```python
from build123d import *

# Parameters (mm, degrees)
F1_DEPTH = 5
F2_DEPTH = 4
F3_DEPTH = 4
F4_R     = 3.22905
F4_R_2   = 3.229051
F5_DEPTH = 25


with BuildPart() as f1:
    # F0 (on Top) → F1 (new body)
    with BuildSketch(Plane.XY):
        Polygon((16.577804, 72.764611), (3.665576, 72.739941), (-9.246652, 72.715272), (-9.147654, 20.899711), (3.838721, 20.904658), (10.953161, 20.92936), (10.913751, 41.556355), (16.625739, 47.675223), align=None)
    extrude(amount=F1_DEPTH)

    # F0 (on Top) → F2 (join)
    with BuildSketch(Plane.XY):
        Polygon((16.577804, 72.764611), (3.665576, 72.739941), (-9.246652, 72.715272), (-9.147654, 20.899711), (3.838721, 20.904658), (10.953161, 20.92936), (10.913751, 41.556355), (16.625739, 47.675223), align=None)
    extrude(amount=F2_DEPTH)

    # F0 (on Top) → F3 (join)
    with BuildSketch(Plane.XY):
        Polygon((16.577804, 72.764611), (3.665576, 72.739941), (-9.246652, 72.715272), (-9.147654, 20.899711), (3.838721, 20.904658), (10.953161, 20.92936), (10.913751, 41.556355), (16.625739, 47.675223), align=None)
    extrude(amount=F3_DEPTH)

    # F4 (on Top) → F5 (cut)
    with BuildSketch(Plane.XY):
        with Locations((10.293464, 47.669735)):
            Circle(F4_R)
        with Locations((11.692577, 68.456538)):
            Circle(F4_R_2)
        with Locations((-4.947346, 68.456538)):
            Circle(F4_R_2)
    extrude(amount=F5_DEPTH, mode=Mode.SUBTRACT)


solid = f1.part
```
Can you work these out from the model? Positions are in its coordinate system, mm. Coordinates: 2 decimals unless noted, no trailing zeros. Order: outer loops, then holes, each group sorted by start corner. A loop starts at its lowest first (then second) coordinate and runs counter-clockwise, first axis right, second up.
1. If we section it at D-D (z = 3.1): Please give me the cut outline in (x, y).
2. If we section it at A-A (x = 12.75): Please give me the cut outline in (y, z), then the cut area to 3 significant figures.
3. If we section it at C-C (y = 50): Please give me the cut outline in (x, z).
4. If we section it at B-B (y = 66): Please give me the cut outline in (x, z).
5. Thinking about a two-plate mould opening in Y: for faces 1 (the face through (1, 47, 5)), 2 (the face through (10.993, 65.304, 2.465)), which applies, +Y half, -Y half, draft (parallel to the pull), parting line (faces both ways), or undercut?
6. I'm going to push a flat-ended pin straight in: pin 1 (2 mm diameter, centred on x = 9, z = 1.5, fed in from +Y). Where does the tip first touch, or does it pass through?
7. I need wall thicknesses on line 1 (X direction, y = 67.5, z = 4.05); line 2 (Y direction, x = 13.25, z = 0.5); line 3 (Y direction, x = 12, z = 3.3). Which ranges of each line are inside material? Lowest first, please.
Entries:
1. outline: (-9.25, 72.72) - (-9.15, 20.9) - (3.84, 20.9) - (10.95, 20.93) - (10.91, 41.56) - (16.63, 47.68) - (16.58, 72.76) - close; hole circle Ø6.46 at (-4.95, 68.46); hole circle Ø6.46 at (10.29, 47.67); hole circle Ø6.46 at (11.69, 68.46)
2. outline: (43.52, 0) - (45.57, 0) - (45.57, 5) - (43.52, 5) - close; (49.77, 0) - (65.41, 0) - (65.41, 5) - (49.77, 5) - close; (71.51, 0) - (72.76, 0) - (72.76, 5) - (71.51, 5) - close
2. area: 94.7 mm2
3. outline: (-9.2, 0) - (8.06, 0) - (8.06, 5) - (-9.2, 5) - close; (12.53, 0) - (16.62, 0) - (16.62, 5) - (12.53, 5) - close
4. outline: (-9.23, 0) - (-7.04, 0) - (-7.04, 5) - (-9.23, 5) - close; (-2.85, 0) - (9.6, 0) - (9.6, 5) - (-2.85, 5) - close; (13.79, 0) - (16.59, 0) - (16.59, 5) - (13.79, 5) - close
5. face 1: draft
5. face 2: undercut
6. pin 1: stops at y = 72.75
7. line 1: x = -9.24 to -8.03, -1.86 to 8.61, 14.78 to 16.59
7. line 2: y = 44.06 to 46.37, 48.97 to 65.63, 71.29 to 72.76
7. line 3: y = 42.72 to 44.93, 50.41 to 65.24, 71.67 to 72.76
